Answer from the drawing. Dimensions are ordinates in mm from the lowest x, y and z of the part. Coordinates: 2 decimals unless noted, no trailing zeros. Write each loop counter-clockwise with the first axis right and the second up, starting at its lowest first coordinate (ties: lowest second). Pieces come first, ordered by that corner, then holes. Notation, with made-up numbers: (67.25, -35) - (94.25, -35) arc R14 ccw to (94.25, -11) - close; hole circle Ø5 at (-16.5, 89). An arc over 180 degrees is marked (long way). Use CSV: the item, a comma, the result in double quotes. Start each with the question number.
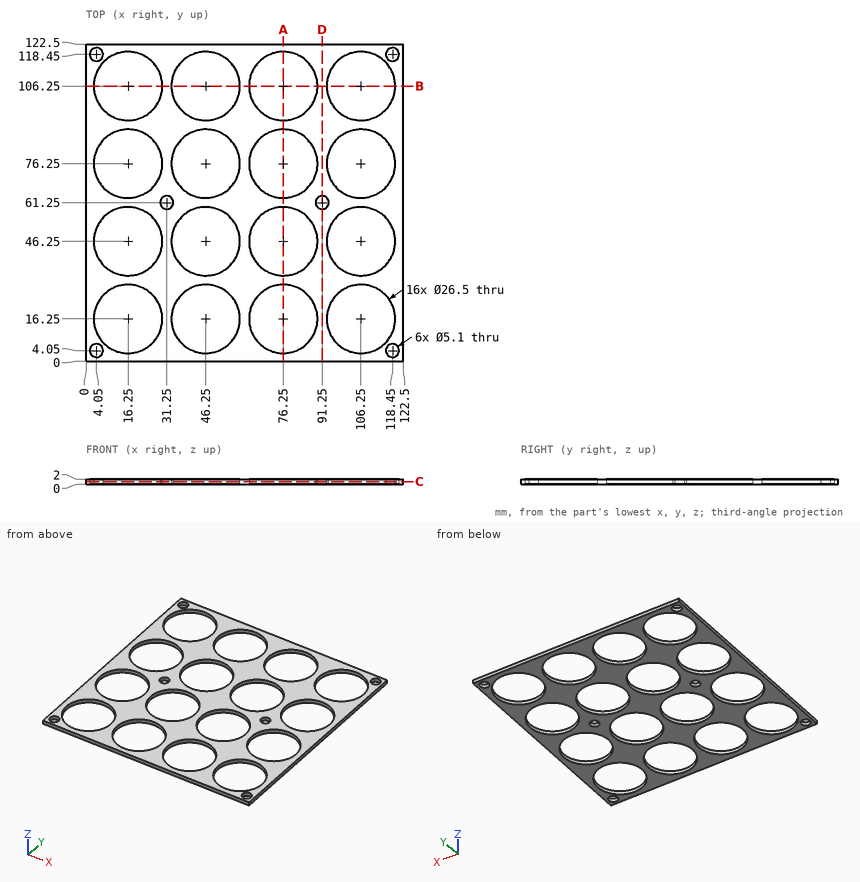
Item 1: A cutting plane is placed at A-A (x = 76.25). Determine the outline of the cut face in (y, z), then the cut area to 3 significant figures.
Item 2: A cutting plane is placed at D-D (x = 91.25). Determine the outline of the cut face in (y, z), then the cut area to 3 significant figures.
Item 3: A cutting plane is placed at C-C (z = 1). Count the separate pieces of the cut face and the enclosed holes in it, then the cut area to 3 significant figures.
Item 4: Each of these flat-tipped pins is pushed along its axis until it touches: pin 1 (6 mm diameter, centred on x = 92.5, y = 35.5, fed in from -Z); pin 2 (24 mm diameter, centred on x = 16.25, y = 76.25, fed in from -Z). Where does it stop, or does it pass through?
Item 5: Straight lines are drawn through the part: probe 1 along Y at (x, z) = (17, 1.9); probe 2 along Y at (x, z) = (71, 1.4); probe 3 along X at (y, z) = (88, 1.85). For each, find the intervals that lie inside material, in ascending order. Write a range as [from, to].
Calculated:
1,outline,"(0, 0) - (3, 0) - (3, 2) - (0, 2) - close; (29.5, 0) - (33, 0) - (33, 2) - (29.5, 2) - close; (59.5, 0) - (63, 0) - (63, 2) - (59.5, 2) - close; (89.5, 0) - (93, 0) - (93, 2) - (89.5, 2) - close; (119.5, 0) - (122.5, 0) - (122.5, 2) - (119.5, 2) - close"
1,area,"33.0 mm²"
2,outline,"(0, 0) - (58.7, 0) - (58.7, 2) - (0, 2) - close; (63.8, 0) - (122.5, 0) - (122.5, 2) - (63.8, 2) - close"
2,area,"235 mm²"
3,separate pieces,"1"
3,enclosed holes,"22"
3,area,"6,060 mm²"
4,pin 1,"stops at z = 0"
4,pin 2,"passes through"
5,probe 1,"y = [0, 3.02], [29.48, 33.02], [59.48, 63.02], [89.48, 93.02], [119.48, 122.5]"
5,probe 2,"y = [0, 4.08], [28.42, 34.08], [58.42, 64.08], [88.42, 94.08], [118.42, 122.5]"
5,probe 3,"x = [0, 10.13], [22.37, 40.13], [52.37, 70.13], [82.37, 100.13], [112.37, 122.5]"
